from build123d import *

# Parameters (mm, degrees)
SKETCH3_R               = 8
BOSS_EXTRUDE1_DEPTH     = 20.490526316
CUT_EXTRUDE1_DEPTH      = 11.102334007
CUT_EXTRUDE1_DEPTH_BACK = 11.102334007
CUT_EXTRUDE2_DEPTH      = 11.089230335
CUT_EXTRUDE2_DEPTH_BACK = 11.089230335
BOSS_EXTRUDE3_DEPTH     = 1.2
SKETCH8_R               = 1.6
SKETCH8_R_2             = 1.4
CUT_EXTRUDE3_DEPTH      = 24.833519451
CUT_EXTRUDE3_DEPTH_BACK = 2.513887999
CUT_EXTRUDE4_DEPTH      = 23.004414315


with BuildPart() as part:
    # Sketch3 → Boss-Extrude1 (new body)
    with BuildSketch(Plane(origin=(-12.082314344, 217.636022384, 0), x_dir=(-0.994665758, -0.103150523, 0), z_dir=(0.103150523, -0.994665758, 0))):
        Circle(SKETCH3_R)
    extrude(amount=BOSS_EXTRUDE1_DEPTH)

    # Sketch4 → Cut-Extrude1 (cut, two sides)
    with BuildSketch(Plane(origin=(10.375761543, 1.076004901, 0), x_dir=(0.103150523, -0.994665758, 0), z_dir=(-0.994665758, -0.103150523, 0))) as cut_extrude1_sk:
        with BuildLine():
            Line((-217.721396158, 8), (-213.721396158, 8))
            ThreePointArc((-213.721396158, 8), (-217.59367935, 0), (-213.721396158, -8))
            Line((-213.721396158, -8), (-217.721396158, -8))
            Line((-217.721396158, -8), (-217.721396158, 8))
        make_face()
    extrude(amount=CUT_EXTRUDE1_DEPTH, mode=Mode.SUBTRACT)
    extrude(cut_extrude1_sk.sketch, amount=-CUT_EXTRUDE1_DEPTH_BACK, mode=Mode.SUBTRACT)

    # Sketch5 → Cut-Extrude2 (cut, two sides)
    with BuildSketch(Plane(origin=(10.375761543, 1.076004901, 0), x_dir=(0.103150523, -0.994665758, 0), z_dir=(-0.994665758, -0.103150523, 0))) as cut_extrude2_sk:
        Polygon((-197.230869842, 0), (-205.230869842, 8), (-197.230869842, 8), align=None)
    extrude(amount=CUT_EXTRUDE2_DEPTH, mode=Mode.SUBTRACT)
    extrude(cut_extrude2_sk.sketch, amount=-CUT_EXTRUDE2_DEPTH_BACK, mode=Mode.SUBTRACT)

    # Sketch7 → Boss-Extrude3 (add, symmetric)
    with BuildSketch(Plane(origin=(10.375761543, 1.076004901, 0), x_dir=(0.103150523, -0.994665758, 0), z_dir=(-0.994665758, -0.103150523, 0))):
        with BuildLine():
            Line((-199.210768829, 1.979898987), (-197.230869842, 0))
            Line((-197.230869842, 0), (-197.230869842, -2.8))
            Line((-197.230869842, -2.8), (-194.805998711, 1.4))
            ThreePointArc((-194.805998711, 1.4), (-196.865396504, 2.776045612), (-199.210768829, 1.979898987))
        make_face()
    extrude(amount=BOSS_EXTRUDE3_DEPTH, both=True)

    # Sketch8 → Cut-Extrude3 (cut, two sides)
    with BuildSketch(Plane(origin=(-12.082314344, 217.636022384, 0), x_dir=(-0.994665758, -0.103150523, 0), z_dir=(0.103150523, -0.994665758, 0))) as cut_extrude3_sk:
        with Locations((-3.6, 3)):
            Circle(SKETCH8_R)
        with Locations((3.6, 3)):
            Circle(SKETCH8_R)
        with Locations((0, -5.5)):
            Circle(SKETCH8_R_2)
    extrude(amount=CUT_EXTRUDE3_DEPTH, mode=Mode.SUBTRACT)
    extrude(cut_extrude3_sk.sketch, amount=-CUT_EXTRUDE3_DEPTH_BACK, mode=Mode.SUBTRACT)

    # Sketch9 → Cut-Extrude4 (cut, through all)
    with BuildSketch(Plane(origin=(-20.344467381, 196.178792599, 0), x_dir=(0.994665758, 0.103150523, 0), z_dir=(0.103150523, -0.994665758, 0))):
        with BuildLine():
            Line((7.933405986, -7.6), (12.929404385, -7.6))
            ThreePointArc((12.929404385, -7.6), (10.431405186, -8), (7.933405986, -7.6))
        make_face()
        with BuildLine():
            Line((7.933405986, 7.6), (12.929404385, 7.6))
            ThreePointArc((12.929404385, 7.6), (10.431405186, 8), (7.933405986, 7.6))
        make_face()
    extrude(amount=-CUT_EXTRUDE4_DEPTH, mode=Mode.SUBTRACT)


solid = part.part
For this review, take the finished solid that the model builds, in its own axes (mm). A direction names the side the tool comes from. Round coordinates to 2 decimals unless told otherwise and drop trailing zeros. Write each loop counter-clockwise with the first axis right and the second up, starting at its lowest first coordinate (ties: lowest second). Pieces come first, ordered by that corner, then holes. Notation, with made-up numbers: (-9, 79) - (18, 79) arc R24 cw to (18, 116) - close; hole circle Ø2 at (-18.5, 26). An arc over 180 degrees is marked (long way). Use a Markdown table: item, result.
Q1. We need section A-A (z = -2.5). Give the boundary of the cut face in (x, y), plus the area to 3 significant figures.
Derived:
| item | result |
|---|---|
| outline | (-19.6, 216.42) - (-17.53, 196.47) - (-15.06, 196.73) - (-17.13, 216.67) - close; (-14.11, 216.98) - (-12.04, 197.04) - (-11.16, 197.13) - (-11.14, 196.96) - (-8.76, 197.21) - (-8.78, 197.38) - (-7.9, 197.47) - (-9.97, 217.41) - close; (-6.94, 217.73) - (-4.88, 197.78) - (-2.41, 198.04) - (-4.48, 217.98) - close |
| area | 183 mm2 |
Q2. The part is to be moulded in two halves that separate along X. For faces 4 (the flat face through (-9.862, 196.064, -0.729)), 5 (the cylindrical face through (-14.26, 207.14, -1.44)), 6 (the cylindrical face through (-11.96, 217.52, 0.12)), say which applies: pulls with the +X half, pulls with the -X half, needs draft (parallel to the pull), parting line crosses it, or undercut.
Derived:
| item | result |
|---|---|
| face 4 | pulls with the +X half |
| face 5 | undercut |
| face 6 | pulls with the -X half |
Q3. Wall thickness on line 1 along X through (y, z) = (202.25, -3); line 2 along X through (y, z) = (208.5, -2.75); line 3 along Z through (x, y) = (-7.5, 203.25): over which ranges is each line inside the solid? List them lowest first.
Derived:
| item | result |
|---|---|
| line 1 | x = -17.94 to -15.71, -12.5 to -8.48, -5.26 to -3.03 |
| line 2 | x = -18.69 to -16.34, -13.17 to -9.1, -5.93 to -3.58 |
| line 3 | z = -7.39 to -4.51, -1.49 to 5.71 |
Q4. Machinability: for faces 1 (the flat face through (-8.755, 197.188, 0.661)), 2 (the flat face through (-11.143, 196.94, 0.661)), 3 (the cylindrical face through (-8.18, 207.77, -1.58)), which of the approach directions +Z, -Z, +X, -X, +Y, -Y give a long, thin tool a straight path to every point of the face, cutting with its end or side? Answer none if there is none.
Derived:
| item | result |
|---|---|
| face 1 | +Z, +X |
| face 2 | +Z, -Y |
| face 3 | none |
Q5. Clearance check with flat-ended pins moving along their axes: pin 1 (4 mm diameter, centred on y = 215.5, z = 2.5, fed in from -X); pin 2 (6 mm diameter, centred on x = -16, z = 3, fed in from -Y); pin 3 (2 mm diameter, centred on x = -5, y = 207.5, fed in from +Z); pin 4 (10 mm diameter, centred on x = -10.5, y = 202, fed in from +Z). State where each tip first meets the part, or that it passes through.
Derived:
| item | result |
|---|---|
| pin 1 | stops at x = -19.98 |
| pin 2 | stops at y = 196.61 |
| pin 3 | stops at z = 6.25 |
| pin 4 | stops at z = 7.6 |
Q6. We need section B-B (y = 206). State how many separate pieces and enclosed holes the cut face has, plus the area to 3 significant figures.
Derived:
| item | result |
|---|---|
| separate pieces | 1 |
| enclosed holes | 3 |
| area | 177 mm2 |
Q7. We need section C-C (z = -5.25). Give the boundary of the cut face in (x, y).
Derived:
| item | result |
|---|---|
| outline | (-17.92, 215.44) - (-15.97, 196.63) - (-3.96, 197.88) - (-5.91, 216.68) - close |
